Part model, mm, in its own coordinate system. Face numbers are marked on the shaded views. Coordinates: 2 decimals unless noted, no trailing zeros. Loops run counter-clockwise (first coordinate to the right, second up) from the corner with the lowest first, then second, coordinate; pieces in that order, holes last. Notation, with made-up numbers: (36, -19) - (60, -19) arc R18 ccw to (60, 14) - close; hole circle Ø3 at (44, 40.5). An arc over 180 degrees is marked (long way). Use a Markdown table: item, result. Add a question column.
1. Wall check: probe 1 along Z at (x, y) = (8, -18.5); probe 2 along X at (y, z) = (-20, -7.55); probe 3 along Y at (x, z) = (0.25, 0.5). Give the ranges that are in metal, low to high. Write a range as [from, to].
2. Band-saw the part on C-C, the plane z = -7.55. Give the cut face in (x, y).
3. Band-saw the part on D-D, the plane x = 8. Give the cut face in (y, z), plus the area to 3 significant figures.
4. Pull direction Y, two halves, no side cores. Call the marked faces 1, 2, 3 and 4: pulls with the +Y half, pulls with the -Y half, needs draft (parallel to the pull), parting line crosses it, or undercut.
5. Band-saw the part on A-A, the plane x = 0. Give the cut face in (y, z).
6. Band-saw the part on B-B, the plane z = -14.5. Give the cut face in (x, y), plus the area to 3 significant figures.
7. Drop flat-ended pins along their axis: pin 1 (5 mm diameter, centred on x = -7.5, z = -3.5, fed in from +Y); pin 2 (3 mm diameter, centred on x = 8, z = -7.55, fed in from -Y); pin 3 (9 mm diameter, centred on x = 0, y = 0, fed in from +Z). Give the stop position or say it passes through.
from build123d import *

# Parameters (mm, degrees)
SKETCH_1_R          = 4
SKETCH_1_R_2        = 1.5
EXTRUDE_1_DEPTH     = 3.3
SKETCH_2_W          = 26.5
SKETCH_2_H          = 3.3
EXTRUDE_2_DEPTH     = 29.7
SKETCH_3_R          = 4.9
SKETCH_3_R_2        = 1.65
CUT_EXTRUDE_1_DEPTH = 3.3


with BuildPart() as part:
    # 草图1 → 凸台-拉伸1 (new body)
    with BuildSketch(Plane.XY):
        with BuildLine():
            Line((-13.25, 0), (-13.25, -20.75))
            Line((-13.25, -20.75), (13.25, -20.75))
            Line((13.25, -20.75), (13.25, 0))
            ThreePointArc((13.25, 0), (0, 13.25), (-13.25, 0))
        make_face()
        Circle(SKETCH_1_R, mode=Mode.SUBTRACT)
        with Locations((-8.5, 0)):
            Circle(SKETCH_1_R_2, mode=Mode.SUBTRACT)
        with Locations((8.5, 0)):
            Circle(SKETCH_1_R_2, mode=Mode.SUBTRACT)
    extrude(amount=EXTRUDE_1_DEPTH)

    # 草图2 → 凸台-拉伸2 (add)
    with BuildSketch(Plane.XY):
        with Locations((0, -19.1)):
            Rectangle(SKETCH_2_W, SKETCH_2_H)
    extrude(amount=-EXTRUDE_2_DEPTH)

    # 草图3 → 切除-拉伸1 (cut)
    with BuildSketch(Plane(origin=(0, -17.45, 0), x_dir=(1, 0, 0), z_dir=(0, 1, 0))):
        with Locations((0, 14.5)):
            Circle(SKETCH_3_R)
        with Locations((-8, 21.55)):
            Circle(SKETCH_3_R_2)
        with Locations((-8, 7.55)):
            Circle(SKETCH_3_R_2)
        with Locations((8, 7.55)):
            Circle(SKETCH_3_R_2)
        with Locations((8, 21.55)):
            Circle(SKETCH_3_R_2)
    extrude(amount=-CUT_EXTRUDE_1_DEPTH, mode=Mode.SUBTRACT)


solid = part.part
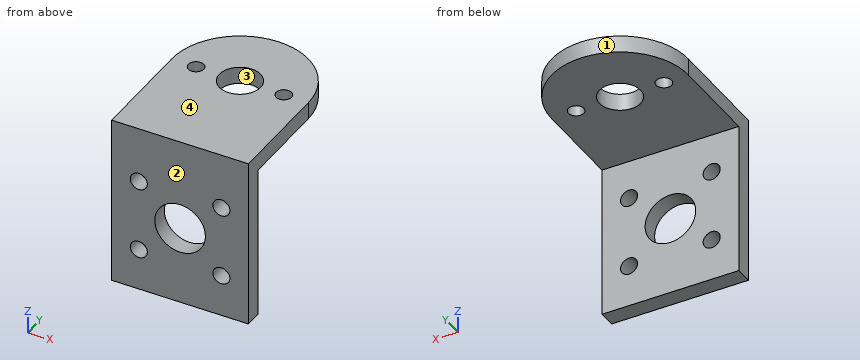
Geometry check:
| question | item | result |
|---|---|---|
| 1 | probe 1 | z = [-29.7, -23.2], [-19.9, -9.2], [-5.9, 3.3] |
| 1 | probe 2 | x = [-13.25, -9.65], [-6.35, 6.35], [9.65, 13.25] |
| 1 | probe 3 | y = [-20.75, -3.99], [3.99, 13.25] |
| 2 | outline | (-13.25, -20.75) - (-9.65, -20.75) - (-9.65, -17.45) - (-13.25, -17.45) - close; (-6.35, -20.75) - (6.35, -20.75) - (6.35, -17.45) - (-6.35, -17.45) - close; (9.65, -20.75) - (13.25, -20.75) - (13.25, -17.45) - (9.65, -17.45) - close |
| 3 | outline | (-20.75, -29.7) - (-17.45, -29.7) - (-17.45, -23.2) - (-20.75, -23.2) - close; (-20.75, -19.9) - (-17.45, -19.9) - (-17.45, -9.2) - (-20.75, -9.2) - close; (-20.75, -5.9) - (-17.45, -5.9) - (-17.45, 0) - (-1.41, 0) - (-1.41, 3.3) - (-20.75, 3.3) - close; (1.41, 0) - (10.56, 0) - (10.56, 3.3) - (1.41, 3.3) - close |
| 3 | area | 170 mm^2 |
| 4 | face 1 | pulls with the +Y half |
| 4 | face 2 | pulls with the -Y half |
| 4 | face 3 | undercut |
| 4 | face 4 | needs draft |
| 5 | outline | (-20.75, -29.7) - (-17.45, -29.7) - (-17.45, -19.4) - (-20.75, -19.4) - close; (-20.75, -9.6) - (-17.45, -9.6) - (-17.45, 0) - (-4, 0) - (-4, 3.3) - (-20.75, 3.3) - close; (4, 0) - (13.25, 0) - (13.25, 3.3) - (4, 3.3) - close |
| 6 | outline | (-13.25, -20.75) - (-4.9, -20.75) - (-4.9, -17.45) - (-13.25, -17.45) - close; (4.9, -20.75) - (13.25, -20.75) - (13.25, -17.45) - (4.9, -17.45) - close |
| 6 | area | 55.1 mm^2 |
| 7 | pin 1 | stops at y = -17.45 |
| 7 | pin 2 | passes through |
| 7 | pin 3 | stops at z = 3.3 |
